Part model, mm, in its own coordinate system. Coordinates: 2 decimals unless noted, no trailing zeros. Order: outer loops, then holes, each group sorted by start corner. A loop starts at its lowest first (then second) coordinate and runs counter-clockwise, first axis right, second up. Notation, with made-up numbers: M 14.25,21.5 L 57.25,21.5 A26 ccw 57.25,58.5 Z; hole C 22.25,-33.75 d10. An arc over 180 degrees is marked long. Write item = value, one per line. Start each with the question number.
from build123d import *

# Parameters (mm, degrees)
SKETCH1_W           = 42.7202667
SKETCH1_H           = 64.4
BOSS_EXTRUDE1_DEPTH = 6.5
SKETCH2_R           = 3.5
CUT_EXTRUDE1_DEPTH  = 7.5
CHAMFER1_SIZE       = 1


with BuildPart() as part:
    # Sketch1 → Boss-Extrude1 (new body)
    with BuildSketch(Plane(origin=(0, 0, 0), x_dir=(1, 0, 0), z_dir=(0, 1, 0))):
        with Locations((-21.36013335, -32.2)):
            Rectangle(SKETCH1_W, SKETCH1_H)
    extrude(amount=BOSS_EXTRUDE1_DEPTH)

    # Sketch2 → Cut-Extrude1 (cut, through all)
    with BuildSketch(Plane(origin=(0, 6.5, 0), x_dir=(1, 0, 0), z_dir=(0, 1, 0))):
        with BuildLine():
            ThreePointArc((-35.690200025, -15.95), (-32.190200025, -19.45), (-28.690200025, -15.95))
            Line((-28.690200025, -15.95), (-35.690200025, -15.95))
        make_face()
        with BuildLine():
            Line((-35.690200025, -15.95), (-28.690200025, -15.95))
            ThreePointArc((-28.690200025, -15.95), (-32.190200025, -12.45), (-35.690200025, -15.95))
        make_face()
        with BuildLine():
            ThreePointArc((-7.030066675, -15.95), (-8.055192941, -13.475126266), (-10.530066675, -12.45))
            Line((-10.530066675, -12.45), (-10.530066675, -15.95))
            Line((-10.530066675, -15.95), (-7.030066675, -15.95))
        make_face()
        with BuildLine():
            Line((-10.530066675, -15.95), (-10.530066675, -12.45))
            ThreePointArc((-10.530066675, -12.45), (-13.004940409, -13.475126266), (-14.030066675, -15.95))
            Line((-14.030066675, -15.95), (-10.530066675, -15.95))
        make_face()
        with BuildLine():
            Line((-7.030066675, -15.95), (-10.530066675, -15.95))
            Line((-10.530066675, -15.95), (-10.530066675, -19.45))
            ThreePointArc((-10.530066675, -19.45), (-8.055192941, -18.424873734), (-7.030066675, -15.95))
        make_face()
        with BuildLine():
            Line((-10.530066675, -19.45), (-10.530066675, -15.95))
            Line((-10.530066675, -15.95), (-14.030066675, -15.95))
            ThreePointArc((-14.030066675, -15.95), (-13.004940409, -18.424873734), (-10.530066675, -19.45))
        make_face()
        with Locations((-32.190200025, -48.45)):
            Circle(SKETCH2_R)
        with BuildLine():
            ThreePointArc((-7.030066675, -48.45), (-8.055192941, -45.975126266), (-10.530066675, -44.95))
            Line((-10.530066675, -44.95), (-10.530066675, -51.95))
            ThreePointArc((-10.530066675, -51.95), (-8.055192941, -50.924873734), (-7.030066675, -48.45))
        make_face()
        with BuildLine():
            Line((-10.530066675, -51.95), (-10.530066675, -44.95))
            ThreePointArc((-10.530066675, -44.95), (-14.030066675, -48.45), (-10.530066675, -51.95))
        make_face()
    extrude(amount=-CUT_EXTRUDE1_DEPTH, mode=Mode.SUBTRACT)

    # Chamfer1
    chamfer1_edges = [part.edges().sort_by_distance(p)[0] for p in [
        (-10.530066675, 6.5, 44.95),
        (-35.690200025, 6.5, 48.45),
        (-28.690200025, 6.5, 15.95),
        (-10.530066675, 6.5, 12.45),
    ]]
    chamfer(chamfer1_edges, length=CHAMFER1_SIZE)


solid = part.part
Item 1: Cut at A-A, the plane y = 4.5. Write the cut outline in (x, z).
Item 2: Cut at B-B, the plane x = -34. Count the separate pieces of the cut face and the enclosed holes in it, and give its area (3 significant figures).
Item 3: Pull direction X, two halves, no side cores. Call faces 1 (the cylindrical face through (-30.575, 2.788, 51.555)), 2 (the flat face through (-22, 3, 0)), 3 (the cylindrical face through (-28.957, 2.788, 17.291)), 4 (the flat face through (0, 3, 33)): pulls with the +X half, pulls with the -X half, needs draft (parallel to the pull), parting line crosses it, or undercut.
Item 4: Wall check: line 1 along X through (y, z) = (1.4, 15.95); line 2 along Z through (x, y) = (-13, 2.75); line 3 along Z through (x, y) = (-12.5, 1.25). Give the ranges that are in metal, low to high. Write a range as [from, to].
Filled sheet:
q1.outline = M -42.72,0 L 0,0 L 0,64.4 L -42.72,64.4 Z; hole C -32.19,15.95 d7; hole C -32.19,48.45 d7; hole C -10.53,15.95 d7; hole C -10.53,48.45 d7
q2.separate_pieces = 3
q2.enclosed_holes = 0
q2.area = 338 mm2
q3.face_1 = undercut
q3.face_2 = needs draft
q3.face_3 = undercut
q3.face_4 = pulls with the +X half
q4.line_1 = [-42.72, -35.69], [-28.69, -14.03], [-7.03, 0]
q4.line_2 = [0, 13.47], [18.43, 45.97], [50.93, 64.4]
q4.line_3 = [0, 13.06], [18.84, 45.56], [51.34, 64.4]
